Part model, mm, in its own coordinate system. Face numbers are marked on the shaded views. A direction names the side the tool comes from. Round coordinates to 2 decimals unless told otherwise and drop trailing zeros. Loops run counter-clockwise (first coordinate to the right, second up) from the corner with the lowest first, then second, coordinate; pieces in that order, holes last.
(1) Cut at D-D on y = 23. List the corners of the cut face in (x, z), then the cut area to 3 significant figures.
(2) Cut at C-C on z = 2.5. List the corners of the cut face in (x, y), then the cut area to 3 significant figures.
(3) Probe probe 1 along X at (y, z) = (-18, 11); probe 2 along Y at (x, z) = (-30, 7.5); probe 3 along Y at (x, z) = (-12.5, 14.75). List the from-to ranges inside material, lowest first.
(4) Flat gauge pins, fed straight in: pin 1 (4 mm diameter, centred on x = -58, y = 0.5, fed in from -Z); pin 2 (2.5 mm diameter, centred on x = -91, y = 14, fed in from -Z); pin 3 (6 mm diameter, centred on y = 10.5, z = 7.5, fed in from -X); pin 4 (4.5 mm diameter, centred on x = -6.33, y = -4.98, fed in from -Z). Where does each tip first touch, or does it go through?
(5) Mould opens along Y. For the marked faces 1, 2 and 3 say: +Y half, -Y half, draft (parallel to the pull), parting line (faces both ways), or undercut.
(6) Cut at B-B on x = 29.5. List the corners of the cut face in (y, z).
(7) Cut at A-A on y = 15.5. List the corners of the cut face in (x, z), then the cut area to 3 significant figures.
(8) Tool access for the marked faces 4 and 5: list every direction of +Z, -Z, +X, -X, +Y, -Y with a clear straight run to the whole face (end or side of a thin tool).
from build123d import *

# Parameters (mm, degrees)
SKETCH_W        = 185
SKETCH_H        = 55
PAD_DEPTH       = 15
SKETCH001_R     = 2.5
SKETCH001_W     = 12
SKETCH001_H     = 16
POCKET_DEPTH    = 5
SKETCH002_W     = 12
SKETCH002_H     = 11
POCKET001_DEPTH = 5
SKETCH003_W     = 180.277405
SKETCH003_H     = 49.743215
POCKET002_DEPTH = 13


with BuildPart() as part:
    # Sketch → Pad (new body)
    with BuildSketch(Plane.XY):
        with Locations((0.0037, 0.153081)):
            Rectangle(SKETCH_W, SKETCH_H)
    extrude(amount=PAD_DEPTH)

    # Sketch001 (on Face6 of Pad) → Pocket (cut)
    with BuildSketch(Plane.XY.offset(15)):
        with Locations((-15.745548, -4.652688)):
            Circle(SKETCH001_R)
        with Locations((-6.327735, -4.978416)):
            Circle(SKETCH001_R)
        with Locations((-16.279421, 10.837662)):
            Rectangle(SKETCH001_W, SKETCH001_H)
    extrude(amount=-POCKET_DEPTH, mode=Mode.SUBTRACT)

    # Sketch002 (on Face1 of Pad) → Pocket001 (cut)
    with BuildSketch(Plane(origin=(-92.4963, 0, 0), x_dir=(0, -1, 0), z_dir=(-1, 0, 0))):
        with Locations((-14.820227, 5.5)):
            Rectangle(SKETCH002_W, SKETCH002_H)
    extrude(amount=-POCKET001_DEPTH, mode=Mode.SUBTRACT)

    # Sketch003 (on Face5 of Pad) → Pocket002 (cut)
    with BuildSketch(Plane(origin=(0, 0, 0), x_dir=(1, 0, 0), z_dir=(0, 0, -1))):
        with Locations((-0.108376, 0.060574)):
            Rectangle(SKETCH003_W, SKETCH003_H)
    extrude(amount=-POCKET002_DEPTH, mode=Mode.SUBTRACT)


solid = part.part
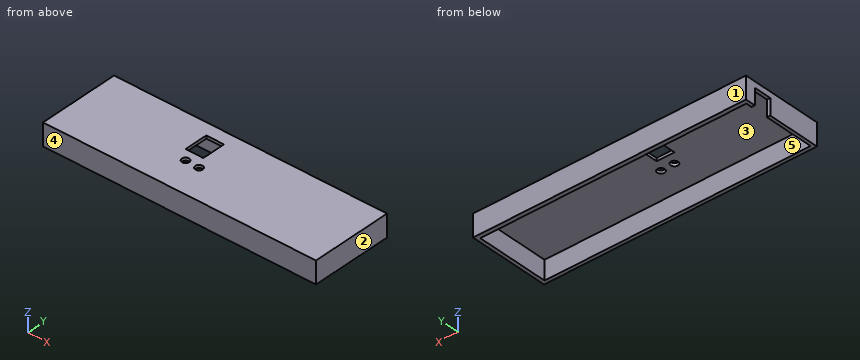
Final values:
1. outline: (-92.5, 0) - (-90.25, 0) - (-90.25, 13) - (90.03, 13) - (90.03, 0) - (92.5, 0) - (92.5, 15) - (-92.5, 15) - close
1. area: 431 mm2
2. outline: (-92.5, -27.35) - (92.5, -27.35) - (92.5, 27.65) - (-92.5, 27.65) - (-92.5, 20.82) - (-90.25, 20.82) - (-90.25, 24.81) - (90.03, 24.81) - (90.03, -24.93) - (-90.25, -24.93) - (-90.25, 8.82) - (-92.5, 8.82) - close
2. area: 1,180 mm2
3. probe 1: x = -92.5 to -90.25, 90.03 to 92.5
3. probe 2: y = -27.35 to -24.93, 24.81 to 27.65
3. probe 3: y = -27.35 to 2.84, 18.84 to 27.65
4. pin 1: stops at z = 13
4. pin 2: stops at z = 11
4. pin 3: stops at x = -92.5
4. pin 4: passes through
5. face 1: +Y half
5. face 2: draft
5. face 3: undercut
6. outline: (-27.35, 0) - (-24.93, 0) - (-24.93, 13) - (24.81, 13) - (24.81, 0) - (27.65, 0) - (27.65, 15) - (-27.35, 15) - close
7. outline: (-92.5, 11) - (-90.25, 11) - (-90.25, 13) - (-22.28, 13) - (-22.28, 15) - (-92.5, 15) - close; (-10.28, 13) - (90.03, 13) - (90.03, 0) - (92.5, 0) - (92.5, 15) - (-10.28, 15) - close
7. area: 383 mm2
8. face 4: +Z, -Z, +X, -X, -Y
8. face 5: -Z
